Drawing for the job (mm, zero at the part's lowest x, y, z). A direction names the side the tool comes from. Coordinates: 2 decimals unless noted, no trailing zeros. Write each loop counter-clockwise with the first axis right and the second up, starting at its lowest first coordinate (ties: lowest second). Pieces come first, ordered by that corner, then holes. Notation, with made-up numbers: M 64.5,38.25 L 120.5,38.25 A12 ccw 120.5,49.25 Z; hole C 76,40 d7. An arc over 180 degrees is marked long. Use a Markdown table: item, result. Add a question column.
Q1. Pin check, flat tips, straight feed: pin 1 Ø0.5 at (x, z) = (0.5, 21) entering from +Y; pin 2 Ø1 at (y, z) = (33, 6.5) entering from -X; pin 3 Ø3 at (x, z) = (4, 1.5) entering from -Y. Stop position of each tip, or through.
Q2. Tool access for the marked faces 1 and 2: list every direction of +Z, -Z, +X, -X, +Y, -Y with a clear straight run to the whole face (end or side of a thin tool).
Q3. Wall check: L1, parallel to Y at x = 8, z = 1.5; L2, parallel to X at y = 18, z = 5.25; L3, parallel to Z at x = 0.75, y = 33.5. Give the ranges that are in metal, low to high. Write a range as from..to.
Q4. Slice it at C-C on y = 21.5. Write the cut outline in (x, z).
Q5. Slice it at A-A on z = 3.75. Write the cut outline in (x, y).
Q6. Slice it at B-B on x = 6. Write the cut outline in (y, z), then the cut area to 3 significant figures.
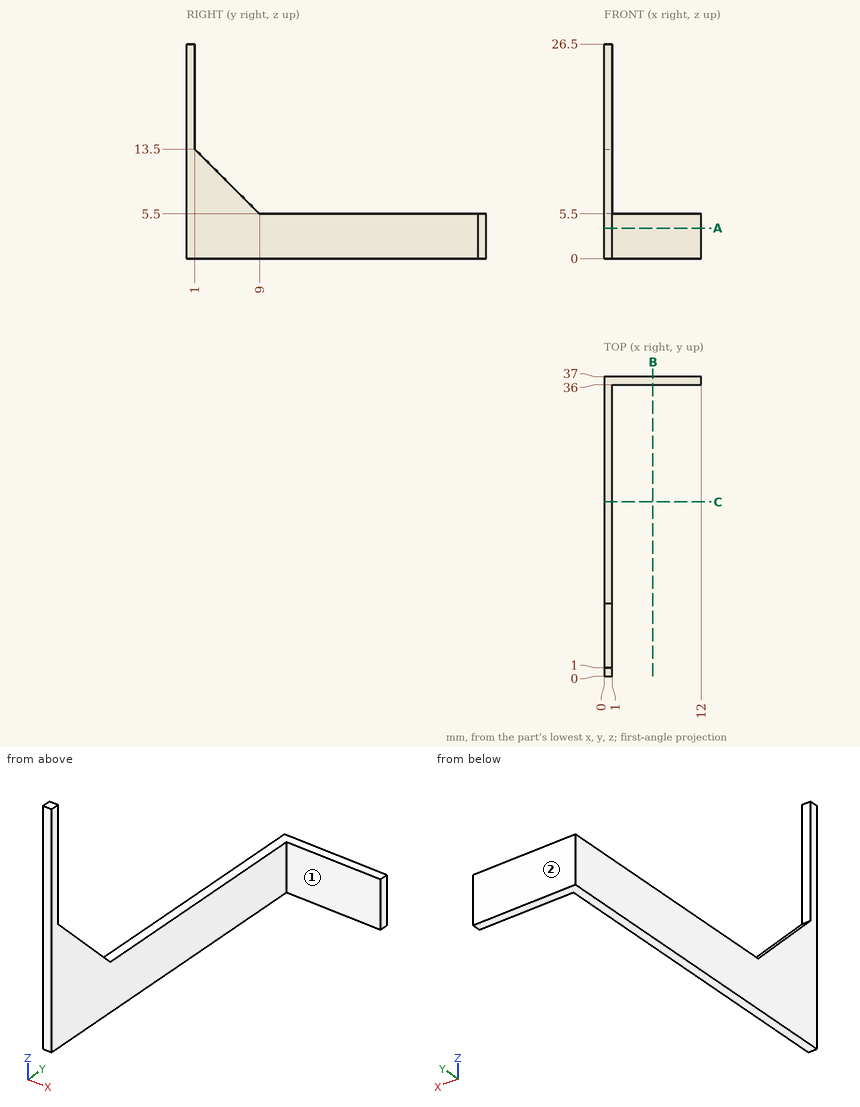
Recorded:
| question | item | result |
|---|---|---|
| 1 | pin 1 | y = 1 |
| 1 | pin 2 | through |
| 1 | pin 3 | y = 36 |
| 2 | face 1 | +Z, -Z, +X, -Y |
| 2 | face 2 | +Z, -Z, +X, -X, +Y |
| 3 | L1 | 36..37 |
| 3 | L2 | 0..1 |
| 3 | L3 | 0..5.5 |
| 4 | outline | M 0,0 L 1,0 L 1,5.5 L 0,5.5 Z |
| 5 | outline | M 0,0 L 1,0 L 1,36 L 12,36 L 12,37 L 0,37 Z |
| 6 | outline | M 36,0 L 37,0 L 37,5.5 L 36,5.5 Z |
| 6 | area | 5.50 mm² |
